```python
from build123d import *

# Parameters (mm, degrees)
SB_BEAM_120_X_12_1_DEPTH = 2000


with BuildPart() as part:
    # Sketch15 → Sb beam 120 X 12(1) (new body)
    with BuildSketch(Plane(origin=(0, 0, 0), x_dir=(-1, 0, 0), z_dir=(0, 1, 0))):
        with BuildLine():
            Line((-30, -60), (-30, -58.080070835))
            ThreePointArc((-30, -58.080070835), (-29.052095223, -55.494589303), (-26.657642624, -54.134502919))
            Line((-26.657642624, -54.134502919), (-9.184714752, -51.222135832))
            ThreePointArc((-9.184714752, -51.222135832), (-4.395809555, -48.501963064), (-2.5, -43.331))
            Line((-2.5, -43.331), (-2.5, 43.331))
            ThreePointArc((-2.5, 43.331), (-4.395809555, 48.501963064), (-9.184714752, 51.222135832))
            Line((-9.184714752, 51.222135832), (-26.657642624, 54.134502919))
            ThreePointArc((-26.657642624, 54.134502919), (-29.052095223, 55.494589303), (-30, 58.080070835))
            Line((-30, 58.080070835), (-30, 60))
            Line((-30, 60), (30, 60))
            Line((30, 60), (30, 58.080070835))
            ThreePointArc((30, 58.080070835), (29.052095223, 55.494589303), (26.657642624, 54.134502919))
            Line((26.657642624, 54.134502919), (9.184714752, 51.222135832))
            ThreePointArc((9.184714752, 51.222135832), (4.395809555, 48.501963064), (2.5, 43.331))
            Line((2.5, 43.331), (2.5, -43.331))
            ThreePointArc((2.5, -43.331), (4.395809555, -48.501963064), (9.184714752, -51.222135832))
            Line((9.184714752, -51.222135832), (26.657642624, -54.134502919))
            ThreePointArc((26.657642624, -54.134502919), (29.052095223, -55.494589303), (30, -58.080070835))
            Line((30, -58.080070835), (30, -60))
            Line((30, -60), (-30, -60))
        make_face()
    extrude(amount=SB_BEAM_120_X_12_1_DEPTH)


solid = part.part
```
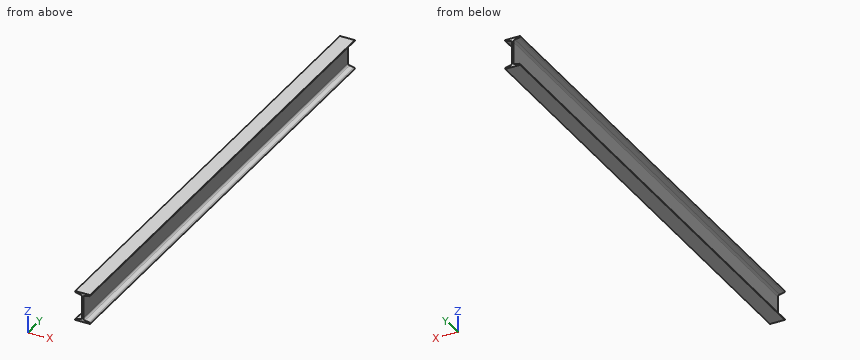
Design review of the part built by this model. Coordinates are the model's own, in mm. Give positions to 0.01 mm unless a question says otherwise; leave off trailing zeros. Loops run counter-clockwise (first coordinate to the right, second up) from the corner with the lowest first, then second, coordinate; pieces in that order, holes last. Notation, with made-up numbers: (-1, -13.5) -> (14, -13.5) arc R35 ccw to (14, 23.5) -> close; hole circle Ø1 at (-7.5, -21.5). An arc over 180 degrees is marked (long way). Write each question's results on one line, items separated by ' | '.
Q1. Wall thickness on L1, parallel to Z at x = -27, y = 96; L2, parallel to Z at x = -8.5, y = 1141.5; L3, parallel to X at y = 1392, z = 37: over which ranges is each line inside the solid? List them lowest first.
Reply:
L1: z = -60 to -54.21, 54.21 to 60 | L2: z = -60 to -51.08, 51.08 to 60 | L3: x = -2.5 to 2.5
Q2. Take a section at A-A, the plane y = 688.5. Write out the cut boundary in (x, z).
Reply:
outline: (-30, -60) -> (30, -60) -> (30, -58.08) arc R4 ccw to (26.66, -54.13) -> (9.18, -51.22) arc R8 cw to (2.5, -43.33) -> (2.5, 43.33) arc R8 cw to (9.18, 51.22) -> (26.66, 54.13) arc R4 ccw to (30, 58.08) -> (30, 60) -> (-30, 60) -> (-30, 58.08) arc R4 ccw to (-26.66, 54.13) -> (-9.18, 51.22) arc R8 cw to (-2.5, 43.33) -> (-2.5, -43.33) arc R8 cw to (-9.18, -51.22) -> (-26.66, -54.13) arc R4 ccw to (-30, -58.08) -> close
Q3. Take a section at B-B, the plane z = -3. Write out the cut boundary in (x, y), plus the area to 3 significant figures.
Reply:
outline: (-2.5, 0) -> (2.5, 0) -> (2.5, 2000) -> (-2.5, 2000) -> close | area: 10,000 mm²
Q4. For pin 1 Ø1 at (x, z) = (4, 34) entering from +Y, flat-tipped, find the tip position at first contact; note if it passes through.
Reply:
pin 1: passes through
